Geometry check sheet. Reference: drawing and pictorial views, mm from the part's lowest x, y, z. A direction names the side the tool comes from. Coordinates: 2 decimals unless noted, no trailing zeros. Loops run counter-clockwise (first coordinate to the right, second up) from the corner with the lowest first, then second, coordinate; pieces in that order, holes last. Notation, with made-up numbers: (69, 8) - (123, 8) arc R10 ccw to (123, 25) - close; hole circle Ø8 at (-17, 28). An arc over 180 degrees is marked (long way). Use a Markdown table: item, result. Add a question column.
1) Draft check along X on the marked faces 1, 2 and 3. Enter one of: pulls with the +X half, pulls with the -X half, needs draft (parallel to the pull), parting line crosses it, or undercut.
2) Sectioned sample at D-D, the plane x = 28.5. Enter the section's corners in (y, z).
3) Thickness scan on line 1 (Y direction, x = 21, z = 8.25); line 2 (Z direction, x = 24.5, y = 13.75); line 3 (X direction, y = 1.5, z = 4). Record the ranges inside material, lowest first.
4) Go/stop test with flat-tipped pins: P1, Ø1, axis at x = 25.5, y = 2.5, coming from the +Z side; P2, Ø6, axis at x = 7.5, y = 6.5, coming from the -Z side. Record where each tip stops, or that it passes through.
5) Sectioned sample at B-B, the plane y = 11.9. Enter the section's corners in (x, z).
6) Tool access check on the marked faces 4 and 5. Record the directions out of +Z, -Z, +X, -X, +Y, -Y that give a thin tool (end or side, any length) a straight path to the whole face; none if there is none.
7) Sectioned sample at A-A, the plane z = 3.25. Enter the section's corners in (x, y), then the cut area to 3 significant figures.
8) Sectioned sample at C-C, the plane x = 3.9. Enter the section's corners in (y, z).
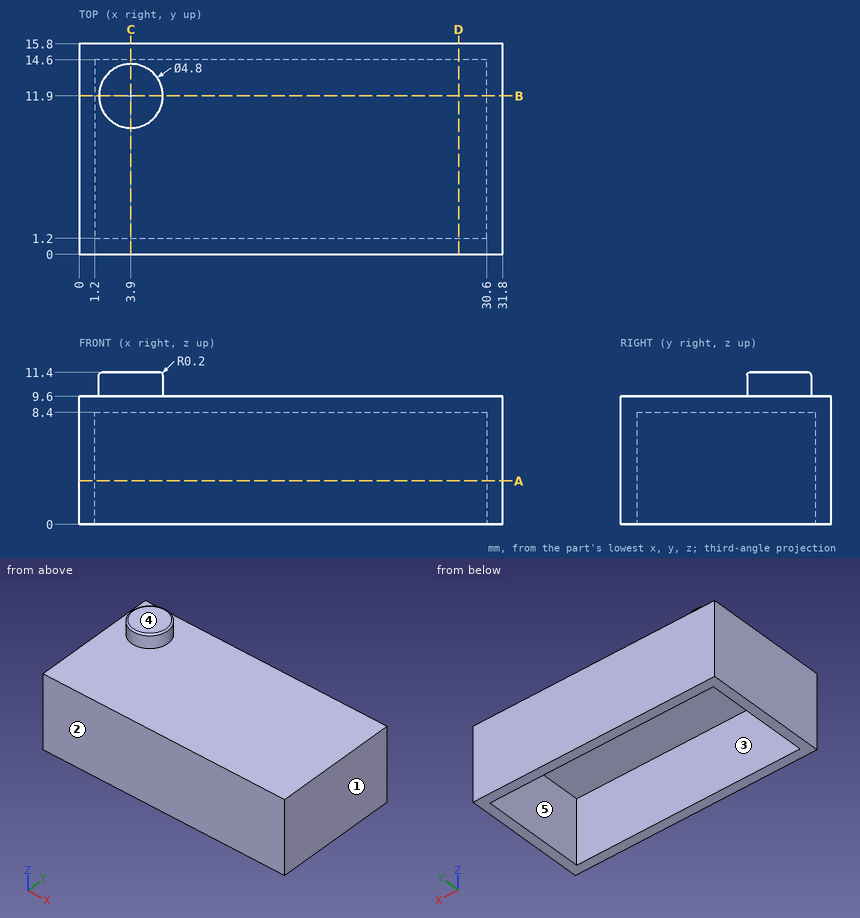
Solved:
| question | item | result |
|---|---|---|
| 1 | face 1 | pulls with the +X half |
| 1 | face 2 | needs draft |
| 1 | face 3 | undercut |
| 2 | outline | (0, 0) - (1.2, 0) - (1.2, 8.4) - (14.6, 8.4) - (14.6, 0) - (15.8, 0) - (15.8, 9.6) - (0, 9.6) - close |
| 3 | line 1 | y = 0 to 1.2, 14.6 to 15.8 |
| 3 | line 2 | z = 8.4 to 9.6 |
| 3 | line 3 | x = 0 to 1.2, 30.6 to 31.8 |
| 4 | P1 | stops at z = 9.6 |
| 4 | P2 | stops at z = 8.4 |
| 5 | outline | (0, 0) - (1.2, 0) - (1.2, 8.4) - (30.6, 8.4) - (30.6, 0) - (31.8, 0) - (31.8, 9.6) - (6.3, 9.6) - (6.3, 11.2) arc R0.2 ccw to (6.1, 11.4) - (1.7, 11.4) arc R0.2 ccw to (1.5, 11.2) - (1.5, 9.6) - (0, 9.6) - close |
| 6 | face 4 | +Z, +X, -X, +Y, -Y |
| 6 | face 5 | -Z |
| 7 | outline | (0, 0) - (31.8, 0) - (31.8, 15.8) - (0, 15.8) - close; hole (1.2, 1.2) - (30.6, 1.2) - (30.6, 14.6) - (1.2, 14.6) - close |
| 7 | area | 108 mm2 |
| 8 | outline | (0, 0) - (1.2, 0) - (1.2, 8.4) - (14.6, 8.4) - (14.6, 0) - (15.8, 0) - (15.8, 9.6) - (14.3, 9.6) - (14.3, 11.2) arc R0.2 ccw to (14.1, 11.4) - (9.7, 11.4) arc R0.2 ccw to (9.5, 11.2) - (9.5, 9.6) - (0, 9.6) - close |
